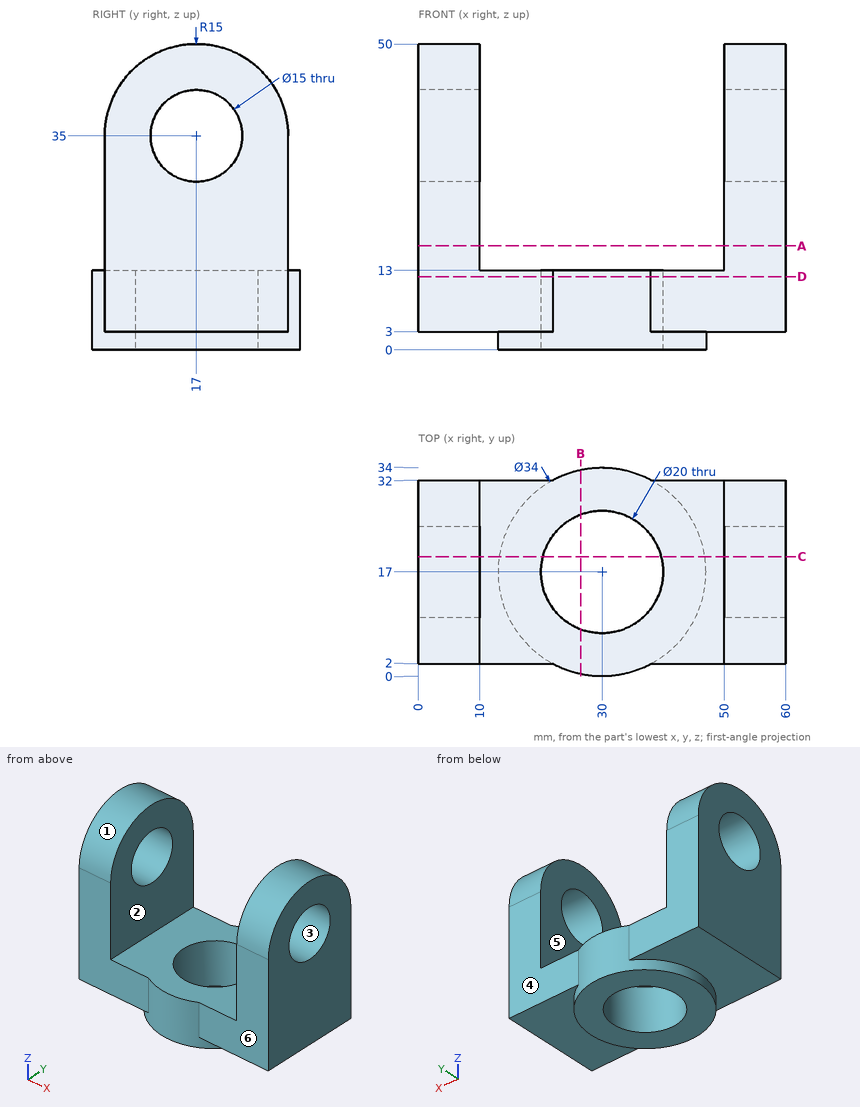
Can you work these out from the drawing? Everything is in mm from the part's minimum corner. A direction names the side the tool comes from. Coordinates: 2 decimals unless noted, no trailing zeros. Loops run counter-clockwise (first coordinate to the right, second up) from the corner with the lowest first, then second, coordinate; pieces in that order, holes last.
1) Will these pins go through, and if not, where does the flat tip stop? pin 1 Ø8 at (x, y) = (51.5, 26) entering from -Z; pin 2 Ø17.5 at (x, z) = (7.5, 17.5) entering from -Y; pin 3 Ø6.5 at (x, z) = (51, 25.5) entering from +Y.
Reported:
pin 1: stops at z = 3
pin 2: stops at y = 2
pin 3: stops at y = 32
2) Imagine slicing it at C-C (y = 19.5). List the corners of the cut face in (x, z) for me.
Reported:
outline: (0, 3) - (13.18, 3) - (13.18, 0) - (20.32, 0) - (20.32, 13) - (10, 13) - (10, 27.93) - (0, 27.93) - close; (0, 42.07) - (10, 42.07) - (10, 49.79) - (0, 49.79) - close; (39.68, 0) - (46.82, 0) - (46.82, 3) - (60, 3) - (60, 27.93) - (50, 27.93) - (50, 13) - (39.68, 13) - close; (50, 42.07) - (60, 42.07) - (60, 49.79) - (50, 49.79) - close
3) Thinking about a two-plate mould opening in Y: for the marked faces 1, 2 and 3, which applies, released by +Y, released by -Y, zero draft, split by the parting line, or undercut?
Reported:
face 1: split by the parting line
face 2: zero draft
face 3: undercut
4) Imagine slicing it at D-D (z = 12). List the corners of the cut face in (x, y) for me, and give its area (3 significant figures).
Reported:
outline: (0, 2) - (22, 2) arc R17 ccw to (38, 2) - (60, 2) - (60, 32) - (38, 32) arc R17 ccw to (22, 32) - (0, 32) - close; hole circle Ø20 at (30, 17)
area: 1,530 mm2
5) Imagine slicing it at A-A (z = 17). List the corners of the cut face in (x, y) for me, and give its area (3 significant figures).
Reported:
outline: (0, 2) - (10, 2) - (10, 32) - (0, 32) - close; (50, 2) - (60, 2) - (60, 32) - (50, 32) - close
area: 600 mm2
6) Which directions (+Z, -Z, +X, -X, +Y, -Y) give clear straight access to the entire face, cutting with the end or side of a thin tool? Please do the marked faces 4, 5 and 6.
Reported:
face 4: +Z, -Z, +X, +Y
face 5: +Z, +Y, -Y
face 6: +Z, -Z, +X, -Y
7) Imagine slicing it at B-B (x = 26.5). List the corners of the cut face in (y, z) for me.
Reported:
outline: (0.36, 0) - (7.63, 0) - (7.63, 13) - (0.36, 13) - close; (26.37, 0) - (33.64, 0) - (33.64, 13) - (26.37, 13) - close
8) Please list where these lines run through material, in increasing order: line 1 along Y through (x, z) = (30, 8.75); line 2 along X through (y, z) = (20, 45); line 3 along Z through (x, y) = (5.75, 17).
Reported:
line 1: y = 0 to 7, 27 to 34
line 2: x = 0 to 10, 50 to 60
line 3: z = 3 to 27.5, 42.5 to 50
